Geometry check sheet. Reference: the model listing, model coordinates, mm. Give positions to 0.01 mm unless a question says otherwise; leave off trailing zeros. Write each loop counter-clockwise with the first axis right and the second up, starting at its lowest first coordinate (ties: lowest second). Pieces come first, ordered by that corner, then holes. Notation, with made-up numbers: M -3.5,-3 L 12.5,-3 A22 ccw 12.5,10 Z; hole C 34,27.5 d7. An arc over 180 degrees is marked long. Write each question's results on one line, items separated by ' | '.
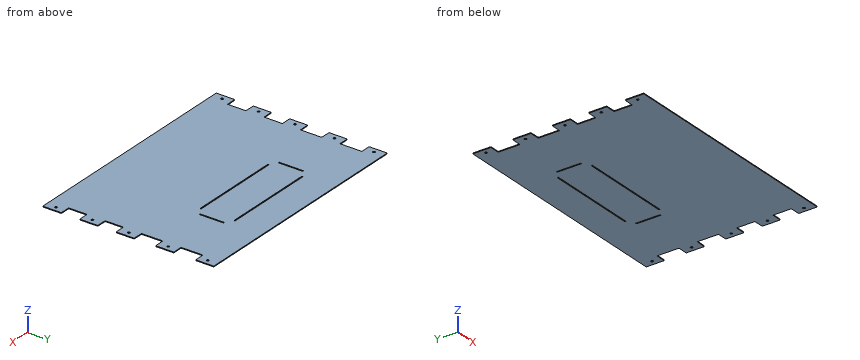
```python
from build123d import *

# Parameters (mm, degrees)
SKETCH1_R           = 3.5
SKETCH1_W           = 271.54175435
SKETCH1_H           = 3.556
SKETCH1_W_2         = 3.556
SKETCH1_H_2         = 71.4883
BOSS_EXTRUDE1_DEPTH = 2.286
FILLET1_R           = 1.27


with BuildPart() as part:
    # Sketch1 → Boss-Extrude1 (new body)
    with BuildSketch(Plane.XY):
        Polygon((-190.471476969, 191.42838219), (503.700363031, 191.42838219), (503.700363031, 138.32838219), (474.617169309, 138.32838219), (474.617169309, 74.041741872), (503.700363031, 74.041741872), (503.700363031, 20.629767615), (474.617169309, 20.629767615), (474.617169309, -42.077913962), (503.700363031, -42.077913962), (503.700363031, -95.085831367), (474.617169309, -95.085831367), (474.617169309, -148.942582796), (503.700363031, -148.942582796), (503.700363031, -201.978007641), (474.617169309, -201.978007641), (474.617169309, -256.009209725), (503.700363031, -256.009209725), (503.700363031, -310.51371781), (-190.471476969, -310.51371781), (-190.471476969, -256.009209725), (-161.388283246, -256.009209725), (-161.388283246, -201.978007641), (-190.471476969, -201.978007641), (-190.471476969, -148.942582796), (-161.388283246, -148.942582796), (-161.388283246, -95.085831367), (-190.471476969, -95.085831367), (-190.471476969, -42.077913962), (-161.388283246, -42.077913962), (-161.388283246, 20.629767615), (-190.471476969, 20.629767615), (-190.471476969, 74.041741872), (-161.388283246, 74.041741872), (-161.388283246, 138.32838219), (-190.471476969, 138.32838219), align=None)
        with Locations((-175.993476969, 163.253382152)):
            Circle(SKETCH1_R, mode=Mode.SUBTRACT)
        with Locations((-175.993476969, 47.335754744)):
            Circle(SKETCH1_R, mode=Mode.SUBTRACT)
        with Locations((-175.993476969, -68.581872664)):
            Circle(SKETCH1_R, mode=Mode.SUBTRACT)
        with Locations((-175.993476969, -175.460295218)):
            Circle(SKETCH1_R, mode=Mode.SUBTRACT)
        with Locations((-175.993476969, -282.338717772)):
            Circle(SKETCH1_R, mode=Mode.SUBTRACT)
        with Locations((489.222363031, 163.253382152)):
            Circle(SKETCH1_R, mode=Mode.SUBTRACT)
        with Locations((489.222363031, 47.335754744)):
            Circle(SKETCH1_R, mode=Mode.SUBTRACT)
        with Locations((489.222363031, -68.581872664)):
            Circle(SKETCH1_R, mode=Mode.SUBTRACT)
        with Locations((489.222363031, -175.460295218)):
            Circle(SKETCH1_R, mode=Mode.SUBTRACT)
        with Locations((489.222363031, -282.338717772)):
            Circle(SKETCH1_R, mode=Mode.SUBTRACT)
        with Locations((157.69971, 98.1583)):
            Rectangle(SKETCH1_W, SKETCH1_H, mode=Mode.SUBTRACT)
        with Locations((-0.762, 47.93615)):
            Rectangle(SKETCH1_W_2, SKETCH1_H_2, mode=Mode.SUBTRACT)
        with Locations((316.16142, 47.93615)):
            Rectangle(SKETCH1_W_2, SKETCH1_H_2, mode=Mode.SUBTRACT)
        with Locations((157.69971, -1.778)):
            Rectangle(SKETCH1_W, SKETCH1_H, mode=Mode.SUBTRACT)
    extrude(amount=BOSS_EXTRUDE1_DEPTH)

    # Fillet1
    fillet1_edges = [part.edges().sort_by_distance(p)[0] for p in [
        (-161.388283246, 74.041741872, 1.143),
        (-161.388283246, 138.32838219, 1.143),
        (-190.471476969, 138.32838219, 1.143),
        (-190.471476969, 191.42838219, 1.143),
        (503.700363031, 191.42838219, 1.143),
        (503.700363031, 138.32838219, 1.143),
        (474.617169309, 138.32838219, 1.143),
        (474.617169309, 74.041741872, 1.143),
        (503.700363031, 74.041741872, 1.143),
        (503.700363031, 20.629767615, 1.143),
        (474.617169309, 20.629767615, 1.143),
        (474.617169309, -42.077913962, 1.143),
        (503.700363031, -42.077913962, 1.143),
        (503.700363031, -95.085831367, 1.143),
        (474.617169309, -95.085831367, 1.143),
        (474.617169309, -148.942582796, 1.143),
        (503.700363031, -148.942582796, 1.143),
        (503.700363031, -201.978007641, 1.143),
        (474.617169309, -201.978007641, 1.143),
        (474.617169309, -256.009209725, 1.143),
        (503.700363031, -256.009209725, 1.143),
        (503.700363031, -310.51371781, 1.143),
        (-190.471476969, -310.51371781, 1.143),
        (-190.471476969, -256.009209725, 1.143),
        (-161.388283246, -256.009209725, 1.143),
        (-161.388283246, -201.978007641, 1.143),
        (-190.471476969, -201.978007641, 1.143),
        (-190.471476969, -148.942582796, 1.143),
        (-161.388283246, -148.942582796, 1.143),
        (-161.388283246, -95.085831367, 1.143),
        (-190.471476969, -95.085831367, 1.143),
        (-190.471476969, -42.077913962, 1.143),
        (-161.388283246, -42.077913962, 1.143),
        (-161.388283246, 20.629767615, 1.143),
        (-190.471476969, 20.629767615, 1.143),
        (-190.471476969, 74.041741872, 1.143),
    ]]
    fillet(fillet1_edges, radius=FILLET1_R)


solid = part.part
```
Q1. Section check B-B (z = 0.4). State how many separate pieces and enclosed holes the cut face has, then the cut area to 3 significant figures.
Answer key:
separate pieces: 1 | enclosed holes: 14 | area: 332,000 mm2
Q2. Material ranges on probe 1 along Y at (x, z) = (109.5, 1.2); probe 2 along X at (y, z) = (21.5, 0.65); probe 3 along X at (y, z) = (-10, 1.1), recorded low to high. Write a range as [from, to].
Answer key:
probe 1: y = [-310.51, -3.56], [0, 96.38], [99.94, 191.43] | probe 2: x = [-190.41, -2.54], [1.02, 314.38], [317.94, 503.64] | probe 3: x = [-161.39, 474.62]
Q3. Section check A-A (y = -226). Enter the section's corners in (x, z).
Answer key:
outline: M -161.39,0 L 474.62,0 L 474.62,2.29 L -161.39,2.29 Z
Q4. Depth check by flat-ended pin: P1, Ø1.1, axis at y = -233.5, z = 1, coming from the -X side; P2, Ø1.5, axis at x = -1.5, y = 50, coming from the -Z side; P3, Ø0.7, axis at y = -223, z = 1.5, coming from the +X side. Enter the tip coordinate at first touch or a pass-through.
Answer key:
P1: stops at x = -161.39 | P2: passes through | P3: stops at x = 474.62
